```python
from build123d import *

# Parameters (mm, degrees)
SKETCH1_W                   = 25.4
SKETCH1_H                   = 25.4
BOSS_EXTRUDE1_DEPTH         = 77.5
M5X0_8_TAPPED_HOLE2_D       = 4.2
M5X0_8_TAPPED_HOLE1_D       = 4.2
M5X0_8_TAPPED_HOLE1_DEPTH   = 10
M5X0_8_TAPPED_HOLE1_TIP     = 1.2618073
SKETCH13_W                  = 25.4
SKETCH13_H                  = 5.5
CUT_EXTRUDE1_DEPTH          = 26.4
TAP_DRILL_FOR_M5X0_8_TAP1_D = 4.2


with BuildPart() as part:
    # Sketch1 → Boss-Extrude1 (new body, symmetric)
    with BuildSketch(Plane.XY):
        Rectangle(SKETCH1_W, SKETCH1_H)
    extrude(amount=BOSS_EXTRUDE1_DEPTH, both=True)

    # M5x0.8 Tapped Hole2 (through all)
    with Locations(Plane(origin=(0, -12.7, 0), x_dir=(-1, 0, 0), z_dir=(0, -1, 0))):
        with Locations((0, -62), (0, 0), (0, 62)):
            Hole(M5X0_8_TAPPED_HOLE2_D / 2)

    # M5x0.8 Tapped Hole1
    with Locations(Plane.XY.offset(77.5)):
        with Locations((0, 0)):
            Hole(M5X0_8_TAPPED_HOLE1_D / 2, depth=M5X0_8_TAPPED_HOLE1_DEPTH)
            with Locations((0, 0, -(M5X0_8_TAPPED_HOLE1_DEPTH + M5X0_8_TAPPED_HOLE1_TIP / 2))):  # 118° drill point
                Cone(0, M5X0_8_TAPPED_HOLE1_D / 2, M5X0_8_TAPPED_HOLE1_TIP, mode=Mode.SUBTRACT)

    # Sketch13 → Cut-Extrude1 (cut, through all)
    with BuildSketch(Plane(origin=(0, 12.7, 0), x_dir=(1, 0, 0), z_dir=(0, 1, 0))):
        with Locations((0, 74.75)):
            Rectangle(SKETCH13_W, SKETCH13_H)
    extrude(amount=-CUT_EXTRUDE1_DEPTH, mode=Mode.SUBTRACT)

    # Tap Drill for M5x0.8 Tap1 (through all)
    with Locations(Plane(origin=(12.7, 0, 0), x_dir=(0, 0, -1), z_dir=(1, 0, 0))):
        with Locations((-49.04, 0), (-18.04, 0), (12.96, 0), (43.96, 0)):
            Hole(TAP_DRILL_FOR_M5X0_8_TAP1_D / 2)


solid = part.part
```
Input: part model. Units: mm. Frame: model coordinates. A direction names the side the tool comes from. Give positions to 0.01 mm unless a question says otherwise; leave off trailing zeros. Order: outer loops, then holes, each group sorted by start corner. A loop starts at its lowest first (then second) coordinate and runs counter-clockwise, first axis right, second up. Notation, with made-up numbers: M 79,43.25 L 115,43.25 A36 cw 115,77.25 Z; hole C 3,48 d9. An arc over 180 degrees is marked long. Return JSON: item names as keys, results as strings.
1) Access query for faces 5 (the face through (0, 0, -72)), 6 (the face through (-2.003, 0.631, 72.43)). Directions: +Z, -Z, +X, -X, +Y, -Y. A direction counts if a zero-diameter tool reaches every point of the face in a straight line with its end or side. Return the directions, or none.
Taken from the geometry:
{"face 5": "-Z, +X, -X, +Y, -Y", "face 6": "+Z"}
2) Mould query, pull axis Z, two halves, no side actions, for faces 1 (the face through (3, 0, 77.5)), 2 (the face through (-1.666, 0.178, -60.722)), 3 (the face through (-12.7, 0, 4)), 4 (the face through (2.003, 0.178, -0.631)). Classes: released by +Z, released by -Z, zero draft, split by the parting line, or undercut.
Taken from the geometry:
{"face 1": "released by +Z", "face 2": "undercut", "face 3": "zero draft", "face 4": "undercut"}
3) Contact query for a flat-ended pin moving along its axis: pin 1 (2.5 mm diameter, centred on y = 0, z = -43.96, fed in from -X). Output: stop coordinate, or through.
Taken from the geometry:
{"pin 1": "passes through"}
4) Section query A-A on z = 18.04. Output: boundary loops of the cut face in (x, y), and give its area (3 significant figures).
Taken from the geometry:
{"outline": "M -12.7,-12.7 L 12.7,-12.7 L 12.7,-2.1 L -12.7,-2.1 Z; M -12.7,2.1 L 12.7,2.1 L 12.7,12.7 L -12.7,12.7 Z", "area": "538 mm2"}
5) Line query: L1, parallel to Z at x = 0.25, y = -2.25; L2, parallel to Y at x = 5.5, z = -12.96. Output: solid intervals per line, ascending. Write a range as [from, to].
Taken from the geometry:
{"L1": "z = [-72, -64.09], [-59.91, -2.09], [2.09, 59.91], [64.09, 77.5]", "L2": "y = [-12.7, -2.1], [2.1, 12.7]"}
